Read the model definition and answer for the solid it produces. Units are mm, in the model's axes. A direction names the side the tool comes from. Coordinates: 2 decimals unless noted, no trailing zeros. Order: outer loops, then holes, each group sorted by start corner. A loop starts at its lowest first (then second) coordinate and runs counter-clockwise, first axis right, second up. Notation, with made-up numbers: M 75.25,42.25 L 85.25,42.25 A7 ccw 85.25,55.25 Z; hole C 85,-8 d5. An arc over 180 degrees is marked long. Put each result on its own line as item: value.
from build123d import *

# Parameters (mm, degrees)
F0_R      = 9.68375
F0_R_2    = 6.50875
F1_DEPTH  = 33.02
F3_DEPTH  = 25
F4_DEPTH  = 54.6
F6_R      = 6.50875
F7_DEPTH  = 3
F9_DEPTH  = 25
F10_DEPTH = 4.9


with BuildPart() as f1:
    # F0 (on Top) → F1 (new body)
    with BuildSketch(Plane.XY):
        Circle(F0_R)
        Circle(F0_R_2, mode=Mode.SUBTRACT)
    extrude(amount=F1_DEPTH)

    # F2 (on Right) → F3 (cut)
    with BuildSketch(Plane.YZ):
        with BuildLine():
            ThreePointArc((7.586009, 0), (0, 7.586009), (-7.586009, 0))
            Line((-7.586009, 0), (7.586009, 0))
        make_face()
    extrude(amount=-F3_DEPTH, mode=Mode.SUBTRACT)

    # F2 (on Right) → F4 (cut)
    with BuildSketch(Plane.YZ):
        with BuildLine():
            ThreePointArc((7.586009, 0), (0, 7.586009), (-7.586009, 0))
            Line((-7.586009, 0), (7.586009, 0))
        make_face()
    extrude(amount=F4_DEPTH, mode=Mode.SUBTRACT)

    # F6 (on offset) → F7 (join)
    with BuildSketch(Plane.XY.offset(20)):
        Circle(F6_R)
    extrude(amount=F7_DEPTH)

    # F8 (on Right) → F9 (cut)
    with BuildSketch(Plane.YZ):
        Polygon((10.249765, 25.931381), (10.093447, 28.872697), (-10.251949, 28.872697), (-10.251949, 25.931381), align=None)
    extrude(amount=-F9_DEPTH, mode=Mode.SUBTRACT)

    # F8 (on Right) → F10 (cut)
    with BuildSketch(Plane.YZ):
        Polygon((10.249765, 25.931381), (10.093447, 28.872697), (-10.251949, 28.872697), (-10.251949, 25.931381), align=None)
    extrude(amount=F10_DEPTH, mode=Mode.SUBTRACT)


solid = f1.part
Q1. Find section C-C on z = 29.5. Write down the section's boundary in (x, y), plus the area to 3 significant figures.
Answers below:
outline: C 0,0 d19.37; hole C 0,0 d13.02
area: 162 mm^2
Q2. Consider line 1 along Z through (x, y) = (0.5, -8.25); line 2 along Y through (x, z) = (0, 29.75). Determine where each line is inside the solid, lowest interval first.
Answers below:
line 1: z = 0 to 25.93, 28.87 to 33.02
line 2: y = -9.68 to -6.51, 6.51 to 9.68
Q3. Find section A-A on y = 0. Write down the section's boundary in (x, z).
Answers below:
outline: M -9.68,7.59 L -6.51,7.59 L -6.51,20 L 6.51,20 L 6.51,7.59 L 9.68,7.59 L 9.68,33.02 L 6.51,33.02 L 6.51,23 L -6.51,23 L -6.51,25.93 L -9.68,25.93 Z; M -9.68,28.87 L -6.51,28.87 L -6.51,33.02 L -9.68,33.02 Z
Q4. Find section B-B on x = 0. Write down the section's boundary in (y, z).
Answers below:
outline: M -9.68,0 L -7.59,0 A7.59 cw -6.51,3.9 L -6.51,20 L 6.51,20 L 6.51,3.9 A7.59 cw 7.59,0 L 9.68,0 L 9.68,25.93 L 6.51,25.93 L 6.51,23 L -6.51,23 L -6.51,25.93 L -9.68,25.93 Z; M -9.68,28.87 L -6.51,28.87 L -6.51,33.02 L -9.68,33.02 Z; M 6.51,28.87 L 9.68,28.87 L 9.68,33.02 L 6.51,33.02 Z
Q5. Given pin 1 (1 mm diameter, centred on y = -1.5, z = 9, fed in from -X); pin 2 (6 mm diameter, centred on x = -5, y = 1.5, fed in from -Z); pin 3 (1.5 mm diameter, centred on x = 1, z = 20, fed in from -Y); pin 4 (10.5 mm diameter, centred on x = -2, y = 3, fed in from -Z), each flat-ended and moving along its own axis, determine where each tip first touches the part or whether it passes through.
Answers below:
pin 1: stops at x = -9.63
pin 2: stops at z = 6.11
pin 3: stops at y = -9.68
pin 4: stops at z = 0
Q6. A tool of negligible diameter and unlimited length cuts with its end or side. For faces 4 (the face through (0, 0, 23)), 5 (the face through (-4.797, 4.399, 13.625)), 6 (the face through (9.237, 2.909, 16.279)), 7 (the face through (4.9, 6, 27)), from which of +Z, -Z, +X, -X, +Y, -Y can it reach the whole face along a straight path? Write none if from no direction.
Answers below:
face 4: +Z
face 5: -Z
face 6: +Z, -Z
face 7: -X, +Y, -Y
Q7. For a pull along Z with two mould halves and no side action, classify faces 1 (the face through (-2.3, -6.3, 33.02)), 2 (the face through (6.208, 1.955, 27.94)), 3 (the face through (4.9, -6, 27)) as +Z half, -Z half, draft (parallel to the pull), parting line (faces both ways), or undercut.
Answers below:
face 1: +Z half
face 2: draft
face 3: undercut
Q8. Find section D-D on y = 3.75. Write down the section's boundary in (x, z), plus the area to 3 significant figures.
Answers below:
outline: M -8.93,6.59 L -5.32,6.59 L -5.32,20 L 5.32,20 L 5.32,6.59 L 8.93,6.59 L 8.93,33.02 L 5.32,33.02 L 5.32,23 L -5.32,23 L -5.32,25.93 L -8.93,25.93 Z; M -8.93,28.87 L -5.32,28.87 L -5.32,33.02 L -8.93,33.02 Z
area: 212 mm^2
